Check sheet for the drawn part. Datum: minimum x, y, z corner. Units: mm. A direction names the side the tool comes from. Round coordinates to 2 decimals unless told otherwise and drop trailing zeros. Loops run counter-clockwise (first coordinate to the right, second up) from the corner with the lowest first, then second, coordinate; pieces in that order, holes last.
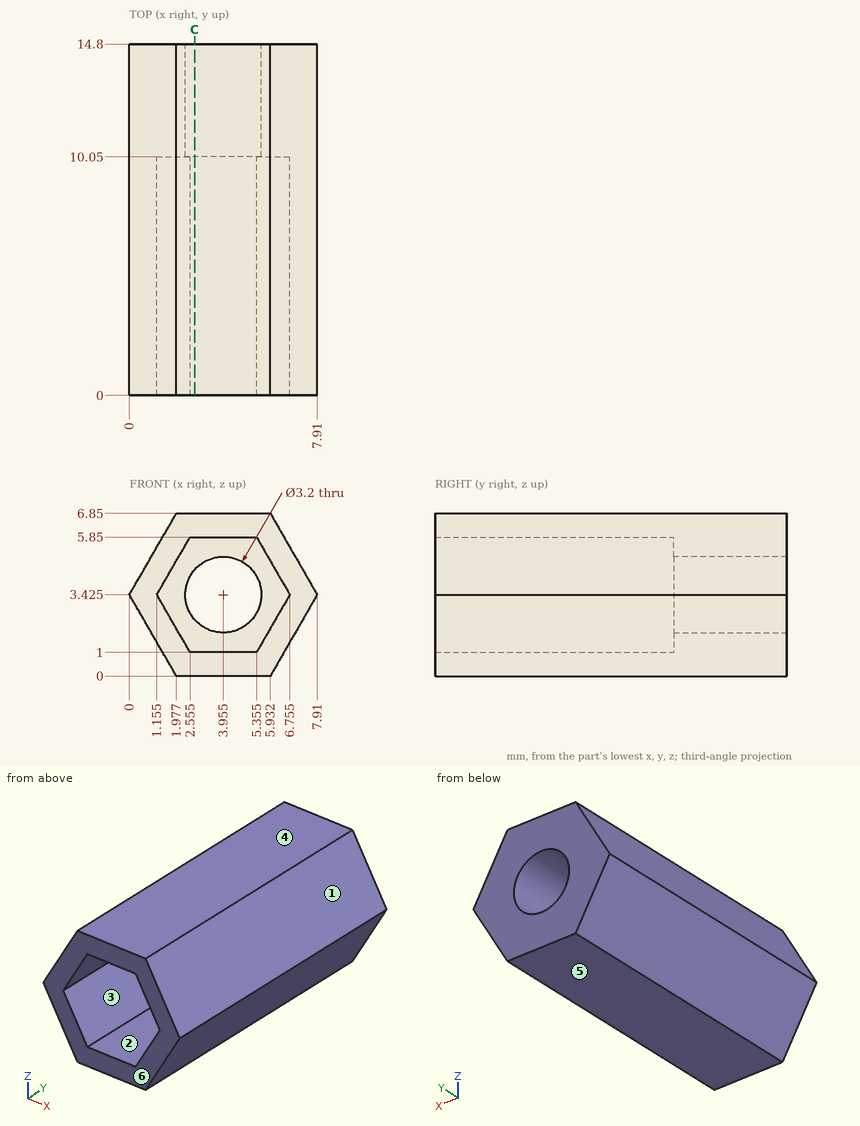
1) Access from +Z, -Z, +X, -X, +Y, -Y to the whole of each face (thin tool, end or side, straight path). Record for the marked faces 1 and 2.
Report:
face 1: +Z, +X, +Y, -Y
face 2: -Y
2) Mould release check, pull along Z, two halves, no side actions. Record for the marked faces 3, 4, 5 and 6: +Z half, -Z half, draft (parallel to the pull), parting line (faces both ways), or undercut.
Report:
face 3: undercut
face 4: +Z half
face 5: -Z half
face 6: draft
3) Sectioned sample at C-C, the plane x = 2.75. Record the cut outline in (y, z).
Report:
outline: (0, 0) - (14.8, 0) - (14.8, 2.37) - (10.05, 2.37) - (10.05, 1) - (0, 1) - close; (0, 5.85) - (10.05, 5.85) - (10.05, 4.48) - (14.8, 4.48) - (14.8, 6.85) - (0, 6.85) - close
4) Gauge pin test, flat end, axial feed: pin 1 (4 mm diameter, centred on y = 10.5, z = 5.5, fed in from -X). Record the tip position at first contact, or that the pin passes through.
Report:
pin 1: stops at x = 0.04
5) Scan lines: line 1 along Z through (x, y) = (2.75, 10); line 2 along Z through (x, y) = (1.75, 4.25) (1 decimal); line 3 along Y through (x, z) = (2.5, 4.5). Record each from-to range of solid material in increasing order.
Report:
line 1: z = 0 to 1, 5.85 to 6.85
line 2: z = 0.4 to 2.4, 4.5 to 6.5
line 3: y = 10.05 to 14.8
